Check sheet for the modelled part. Datum: model origin and axes. Units: mm. A direction names the side the tool comes from. Give positions to 0.01 mm unless a question says otherwise; leave off trailing zeros. Loops run counter-clockwise (first coordinate to the right, second up) from the corner with the lowest first, then second, coordinate; pieces in that order, holes last. Notation, with made-up numbers: (78, 51) -> (116, 51) arc R25 ccw to (116, 82) -> close; hole circle Ø3 at (59, 16.5). An arc over 180 degrees is marked (long way). Answer as CSV lines item,"result". Start each with the question number.
(1) Section check C-C on x = -5. Enter the section's corners in (y, z), plus the area to 3 significant figures.
(2) Material ranges on line 1 (Z direction, x = -3.35, y = 0); line 2 (X direction, y = -2.25, z = -11) (3 decimals); line 3 (X direction, y = 2.5, z = -2.5), recorded low to high. Write a range as from..to.
(3) Section check D-D on y = 10.5. State how many separate pieces and enclosed holes the cut face has, plus the area to 3 significant figures.
(4) Release check for a two-part mould opening along X. For faces 1 (the face through (0, 4, -9)), 2 (the face through (-1.565, 8.736, 3.571)), 3 (the face through (-4.445, -8, 6)) record: pulls with the +X half, pulls with the -X half, needs draft (parallel to the pull), parting line crosses it, or undercut.
(5) Gauge pin test, flat ends, axial feed: pin 1 Ø1.1 at (x, y) = (-2, -11) entering from +Z; pin 2 Ø12 at (y, z) = (1.5, 2) entering from +X; pin 3 Ø8 at (x, z) = (-7.5, 4.5) entering from +Y. Record the tip position at first contact, or that the pin passes through.
(6) Access from +Z, -Z, +X, -X, +Y, -Y to the whole of each face (thin tool, end or side, straight path). Record for faces 4 (the face through (-1.565, -8.248, -6.452)), 5 (the face through (-2.254, -4.418, 10.656)), 6 (the face through (-2, 10, -1.274)), 7 (the face through (-21.826, 9, 5)).
from build123d import *

# Parameters (mm, degrees)
F0_W     = 1.2712626288
F0_H     = 9.6255521612
F3_SIZE  = 1.27
F4_R     = 0.254
F5_DEPTH = 3.175
F6_R     = 9.3595697084
F7_DEPTH = 0.635


with BuildPart() as f1:
    # F0 (on Front) → F1 (revolve)
    with BuildSketch(Plane.XZ):
        Polygon((-15.8015552493, 0), (0, 0), (0, 11.5354972151), (-4.445, 11.5354972151), (-4.445, 9.6304972151), (-6.35, 9.6304972151), (-6.35, 7.7254972151), (-15.8015552493, 9.6255521612), align=None)
        with Locations((-16.4371865637, 4.8127760806)):
            Rectangle(F0_W, F0_H)
        with BuildLine():
            Line((-25.4, 0), (-17.0728178781, 0))
            Line((-17.0728178781, 0), (-17.0728178781, 9.6255521612))
            Line((-17.0728178781, 9.6255521612), (-17.0728178781, 9.8811152703))
            ThreePointArc((-17.0728178781, 9.8811152703), (-19.4495251043, 11.6341692899), (-21.8262323304, 9.8811152703))
            Line((-21.8262323304, 9.8811152703), (-21.8262323304, 12.7))
            Line((-21.8262323304, 12.7), (-25.4, 12.7))
            Line((-25.4, 12.7), (-25.4, 0))
        make_face()
    revolve(axis=Axis((-12.7, 0, 0), (-1, 0, 0)))

    # F3
    f3_edges = [f1.edges().sort_by_distance(p)[0] for p in [
        (-21.826232, 0, -12.7),
    ]]
    chamfer(f3_edges, length=F3_SIZE)

    # F4
    f4_edges = [f1.edges().sort_by_distance(p)[0] for p in [
        (-6.35, 0, -9.630497),
    ]]
    fillet(f4_edges, radius=F4_R)

    # F2 (on face) → F5 (cut)
    with BuildSketch(Plane.YZ):
        with BuildLine():
            ThreePointArc((-7.5107795932, 5.714728369), (-6.6734522711, 6.6734522711), (-5.714728369, 7.5107795932))
            Line((-5.714728369, 7.5107795932), (-7.2092179392, 9.0052691634))
            ThreePointArc((-7.2092179392, 9.0052691634), (-8.1568283052, 8.1568283052), (-9.0052691634, 7.2092179392))
            Line((-9.0052691634, 7.2092179392), (-7.5107795932, 5.714728369))
        make_face()
        with BuildLine():
            ThreePointArc((-1.2562011473, 9.3537099114), (0.0090057319, 9.4376824129), (1.2740500488, 9.3512954665))
            Line((1.2740500488, 9.3512954665), (1.2760667257, 11.464700158))
            ThreePointArc((1.2760667257, 11.464700158), (0.0010145552, 11.5354971705), (-1.2740500488, 11.4649244426))
            Line((-1.2740500488, 11.4649244426), (-1.2562011473, 9.3537099114))
        make_face()
        with BuildLine():
            ThreePointArc((5.714728369, 7.5107795932), (6.6752371757, 6.671666889), (7.5138358891, 5.7107092958))
            Line((7.5138358891, 5.7107092958), (9.0052691634, 7.2092179392))
            ThreePointArc((9.0052691634, 7.2092179392), (8.1568283052, 8.1568283052), (7.2092179392, 9.0052691634))
            Line((7.2092179392, 9.0052691634), (5.714728369, 7.5107795932))
        make_face()
        with BuildLine():
            ThreePointArc((9.3537099114, 1.2562011473), (9.4166691071, 0.6295024673), (9.4376867096, 0))
            ThreePointArc((9.4376867096, 0), (9.4160641292, -0.6384878569), (9.3512954665, -1.2740500488))
            Line((9.3512954665, -1.2740500488), (11.4649244426, -1.2740500488))
            ThreePointArc((11.4649244426, -1.2740500488), (11.517840509, -0.6380015758), (11.5354972151, 0))
            ThreePointArc((11.5354972151, 0), (11.5183888753, 0.6280236595), (11.4671146028, 1.2541844704))
            Line((11.4671146028, 1.2541844704), (9.3537099114, 1.2562011473))
        make_face()
        with BuildLine():
            Line((9.0052691634, -7.2092179392), (7.5107795932, -5.714728369))
            ThreePointArc((7.5107795932, -5.714728369), (6.6734522711, -6.6734522711), (5.714728369, -7.5107795932))
            Line((5.714728369, -7.5107795932), (7.2092179392, -9.0052691634))
            ThreePointArc((7.2092179392, -9.0052691634), (8.1568283052, -8.1568283052), (9.0052691634, -7.2092179392))
        make_face()
        with BuildLine():
            Line((1.2541844704, -11.4671146028), (1.2562011473, -9.3537099114))
            ThreePointArc((1.2562011473, -9.3537099114), (-0.0090057319, -9.4376824129), (-1.2740500488, -9.3512954665))
            Line((-1.2740500488, -9.3512954665), (-1.2740500488, -11.4649244426))
            ThreePointArc((-1.2740500488, -11.4649244426), (-0.0099929726, -11.5354928868), (1.2541844704, -11.4671146028))
        make_face()
        with BuildLine():
            Line((-7.2092179392, -9.0052691634), (-5.7192543462, -7.5073337579))
            ThreePointArc((-5.7192543462, -7.5073337579), (-6.6754631322, -6.6714408039), (-7.5107795932, -5.714728369))
            Line((-7.5107795932, -5.714728369), (-9.0052691634, -7.2092179392))
            ThreePointArc((-9.0052691634, -7.2092179392), (-8.1568283052, -8.1568283052), (-7.2092179392, -9.0052691634))
        make_face()
        with BuildLine():
            ThreePointArc((-9.3512954665, -1.2740500488), (-9.4376867096, 0), (-9.3512954665, 1.2740500488))
            Line((-9.3512954665, 1.2740500488), (-11.464700158, 1.2760667257))
            ThreePointArc((-11.464700158, 1.2760667257), (-11.5354971705, 0.0010145552), (-11.4649244426, -1.2740500488))
            Line((-11.4649244426, -1.2740500488), (-9.3512954665, -1.2740500488))
        make_face()
        with BuildLine():
            ThreePointArc((9.3512954665, -1.2740500488), (9.4160641292, -0.6384878569), (9.4376867096, 0))
            ThreePointArc((9.4376867096, 0), (9.4166691071, 0.6295024673), (9.3537099114, 1.2562011473))
            ThreePointArc((9.3537099114, 1.2562011473), (8.7229115577, 3.6028800126), (7.5138358891, 5.7107092958))
            ThreePointArc((7.5138358891, 5.7107092958), (6.6752371757, 6.671666889), (5.714728369, 7.5107795932))
            ThreePointArc((5.714728369, 7.5107795932), (3.6135343658, 8.7185033014), (1.2740500488, 9.3512954665))
            ThreePointArc((1.2740500488, 9.3512954665), (0.0090057319, 9.4376824129), (-1.2562011473, 9.3537099114))
            ThreePointArc((-1.2562011473, 9.3537099114), (-3.6052132558, 8.721947478), (-5.714728369, 7.5107795932))
            ThreePointArc((-5.714728369, 7.5107795932), (-6.6734522711, 6.6734522711), (-7.5107795932, 5.714728369))
            ThreePointArc((-7.5107795932, 5.714728369), (-8.7185033014, 3.6135343658), (-9.3512954665, 1.2740500488))
            ThreePointArc((-9.3512954665, 1.2740500488), (-9.4376867096, 0), (-9.3512954665, -1.2740500488))
            ThreePointArc((-9.3512954665, -1.2740500488), (-8.7185033014, -3.6135343658), (-7.5107795932, -5.714728369))
            ThreePointArc((-7.5107795932, -5.714728369), (-6.6754631322, -6.6714408039), (-5.7192543462, -7.5073337579))
            ThreePointArc((-5.7192543462, -7.5073337579), (-3.6161616786, -8.7174139023), (-1.2740500488, -9.3512954665))
            ThreePointArc((-1.2740500488, -9.3512954665), (-0.0090057319, -9.4376824129), (1.2562011473, -9.3537099114))
            ThreePointArc((1.2562011473, -9.3537099114), (3.6052132558, -8.721947478), (5.714728369, -7.5107795932))
            ThreePointArc((5.714728369, -7.5107795932), (6.6734522711, -6.6734522711), (7.5107795932, -5.714728369))
            ThreePointArc((7.5107795932, -5.714728369), (8.7185033014, -3.6135343658), (9.3512954665, -1.2740500488))
        make_face()
    extrude(amount=-F5_DEPTH, mode=Mode.SUBTRACT)

    # F6 (on face) → F7 (cut)
    with BuildSketch(Plane.YZ.offset(-3.175)):
        Circle(F6_R)
    extrude(amount=-F7_DEPTH, mode=Mode.SUBTRACT)


solid = f1.part
Working result:
1,outline,"circle Ø19.26 at (0, 0)"
1,area,"291 mm^2"
2,line 1,"z = -11.54..-9.36, 9.36..11.54"
2,line 2,"x = -25.4..-21.826, -20.812..-18.087, -4.445..0"
2,line 3,"x = -25.4..-3.81"
3,separate pieces,"3"
3,enclosed holes,"0"
3,area,"116 mm^2"
4,face 1,"pulls with the +X half"
4,face 2,"needs draft"
4,face 3,"undercut"
5,pin 1,"stops at z = 4.89"
5,pin 2,"stops at x = -3.81"
5,pin 3,"stops at y = 11.37"
6,face 4,"-Z, +X"
6,face 5,"+X"
6,face 6,"+X, +Y, -Y"
6,face 7,"none"
